Verification items for this drawing (mm, ordinates from the low corner). A direction names the side the tool comes from. Round coordinates to 2 decimals unless told otherwise and drop trailing zeros. Loops run counter-clockwise (first coordinate to the right, second up) from the corner with the lowest first, then second, coordinate; pieces in that order, holes last. Notation, with made-up numbers: (84.25, -35) -> (139.25, -35) arc R31 ccw to (139.25, -2) -> close; hole circle Ø6 at (0.25, 10.25). An arc over 180 degrees is marked (long way). Use a Markdown table: item, result. Add a question column.
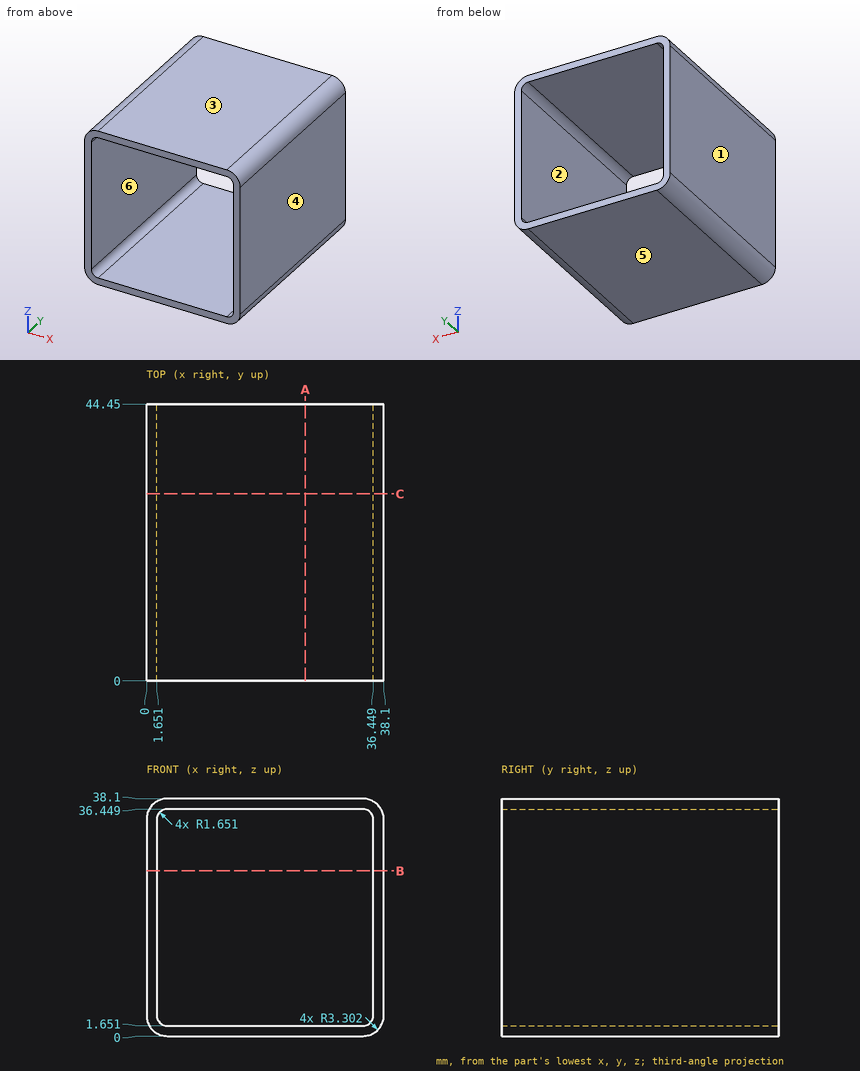
1) Sectioned sample at A-A on x = 25.5. Enter the section's corners in (y, z), then the cut area to 3 significant figures.
2) Release check for a two-part mould opening along Z. For the marked faces 3, 4, 5 and 6 record: released by +Z, released by -Z, zero draft, split by the parting line, or undercut.
3) Thickness scan on line 1 (Z direction, x = 27, y = 19.5); line 2 (X direction, y = 15, z = 36.5). Record the ranges inside material, lowest first.
4) Access from +Z, -Z, +X, -X, +Y, -Y to the whole of each face (thin tool, end or side, straight path). Record for the marked faces 1 and 2.
5) Go/stop test with a flat-tipped pin: pin 1 (12 mm diameter, centred on x = 33.5, y = 26, fed in from -Z). Record where the tip stops, or that it passes through.
6) Sectioned sample at C-C on y = 30. Enter the section's corners in (x, z), then the cut area to 3 significant figures.
7) Sectioned sample at B-B on z = 26.5. Enter the section's corners in (x, y).
Geometry results:
| question | item | result |
|---|---|---|
| 1 | outline | (0, 0) -> (44.45, 0) -> (44.45, 1.65) -> (0, 1.65) -> close; (0, 36.45) -> (44.45, 36.45) -> (44.45, 38.1) -> (0, 38.1) -> close |
| 1 | area | 147 mm^2 |
| 2 | face 3 | released by +Z |
| 2 | face 4 | zero draft |
| 2 | face 5 | released by -Z |
| 2 | face 6 | undercut |
| 3 | line 1 | 0 to 1.65, 36.45 to 38.1 |
| 3 | line 2 | 0.47 to 37.63 |
| 4 | face 1 | +Z, -Z, -X, +Y, -Y |
| 4 | face 2 | +Y, -Y |
| 5 | pin 1 | z = 0 |
| 6 | outline | (0, 3.3) arc R3.3 ccw to (3.3, 0) -> (34.8, 0) arc R3.3 ccw to (38.1, 3.3) -> (38.1, 34.8) arc R3.3 ccw to (34.8, 38.1) -> (3.3, 38.1) arc R3.3 ccw to (0, 34.8) -> close; hole (1.65, 3.3) arc R1.65 ccw to (3.3, 1.65) -> (34.8, 1.65) arc R1.65 ccw to (36.45, 3.3) -> (36.45, 34.8) arc R1.65 ccw to (34.8, 36.45) -> (3.3, 36.45) arc R1.65 ccw to (1.65, 34.8) -> close |
| 6 | area | 234 mm^2 |
| 7 | outline | (0, 0) -> (1.65, 0) -> (1.65, 44.45) -> (0, 44.45) -> close; (36.45, 0) -> (38.1, 0) -> (38.1, 44.45) -> (36.45, 44.45) -> close |
